The figure shows three views and two pictorial views of one solid part (mm, origin at its lowest corner). Answer the questions. A direction names the side the tool comes from. Coordinates: 2 decimals unless noted, no trailing zeros. Order: outer loops, then holes, each group sorted by start corner. A loop starts at its lowest first (then second) coordinate and runs counter-clockwise, first axis right, second up. Notation, with made-up numbers: M 50,46 L 82,46 A29 ccw 82,80 Z; hole C 25.25,36 d7. An arc over 180 degrees is marked long. Answer in a Markdown table with one row per item. Add a question column.
Item 1: Which of the six approach directions +Z, -Z, +X, -X, +Y, -Y give full straight-line access (tool end or side, diameter ignored) to the marked faces 1, 2, 3, 4 and 5?
Item 2: Flat-ended cylindrical pins translate along their axes: pin 1 Ø1 at (x, z) = (204.5, 503) entering from +Y; pin 2 Ø5 at (x, y) = (236.5, 55) entering from -Z (1 decimal); pin 3 Ø10 at (y, z) = (128.5, 486.5) entering from -X. Find the tip coordinate at first contact, or state that the pin passes through.
Item 3: Consider line 1 (X direction, y = 143.5, z = 152) (1 decimal); line 2 (X direction, y = 214, z = 495) (1 decimal); line 3 (Y direction, x = 229, z = 390.5) (1 decimal). Determine where each line is inside the solid, lowest interval first. Write a range as from..to.
Item 4: The part is cut by section C-C (z = 423.5). Write down the section's boundary in (x, y).
Item 5: The part is cut by section B-B (z = 337). Write down the section's boundary in (x, y).
Item 6: The part is cut by section A-A (z = 174.5). Write down the section's boundary in (x, y) (1 decimal), then the cut area to 3 significant figures.
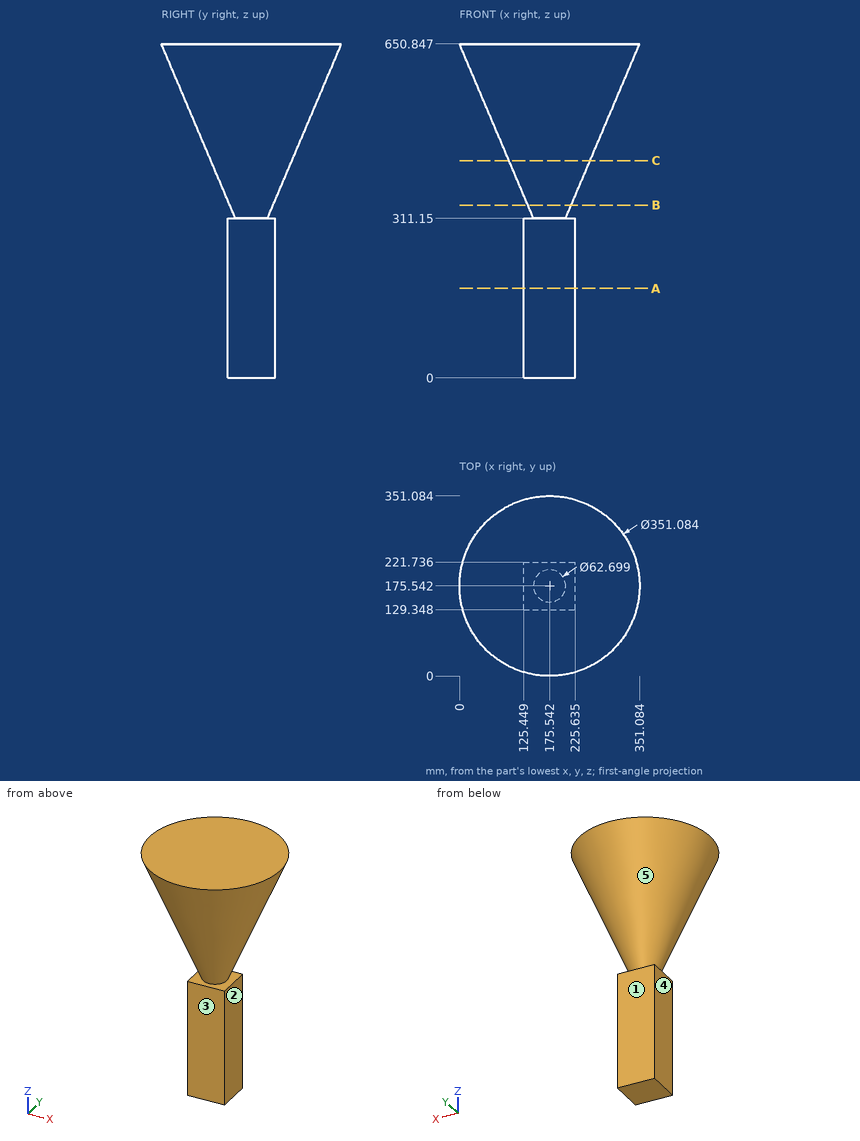
Reply:
| question | item | result |
|---|---|---|
| 1 | face 1 | -Z, +X, -X, +Y |
| 1 | face 2 | -Z, +X, +Y, -Y |
| 1 | face 3 | -Z, +X, -X, -Y |
| 1 | face 4 | -Z, -X, +Y, -Y |
| 1 | face 5 | none |
| 2 | pin 1 | stops at y = 284.8 |
| 2 | pin 2 | stops at z = 549.6 |
| 2 | pin 3 | stops at x = 77.48 |
| 3 | line 1 | x = 125.4..225.6 |
| 3 | line 2 | x = 73.1..277.9 |
| 3 | line 3 | y = 138.5..212.6 |
| 4 | outline | C 175.54,175.54 d158.08 |
| 5 | outline | C 175.54,175.54 d84.64 |
| 6 | outline | M 125.4,129.3 L 225.6,129.3 L 225.6,221.7 L 125.4,221.7 Z |
| 6 | area | 9,260 mm2 |
